The drawing under review shows one solid part. Ordinate dimensions are in mm from its lowest x, y, z. Round coordinates to 2 decimals unless told otherwise and drop trailing zeros. Write each loop counter-clockwise with the first axis right and the second up, starting at its lowest first coordinate (ties: lowest second). Pieces come first, ordered by that corner, then holes.
Item 1: Clearance check with flat-ended pins moving along their axes: pin 1 Ø1.5 at (x, y) = (11.5, 10) entering from +Z; pin 2 Ø1 at (x, y) = (15, 17) entering from +Z; pin 3 Ø4 at (y, z) = (7, 32.5) entering from +X. State where each tip first meets the part, or that it passes through.
Item 2: Add section A-A (x = 13.5). Give the boundary of the cut face in (y, z).
Item 3: Add section B-B (y = 8.5). Give the boundary of the cut face in (x, z) (1 decimal).
Item 4: To check wall thickness, follow L1, parallel to Y at x = 9, z = 10 (1 decimal); L2, parallel to Y at x = 5.25, z = 62.5; L3, parallel to X at y = 13.75, z = 27. State the ranges of each line that lie inside material, in increasing order.
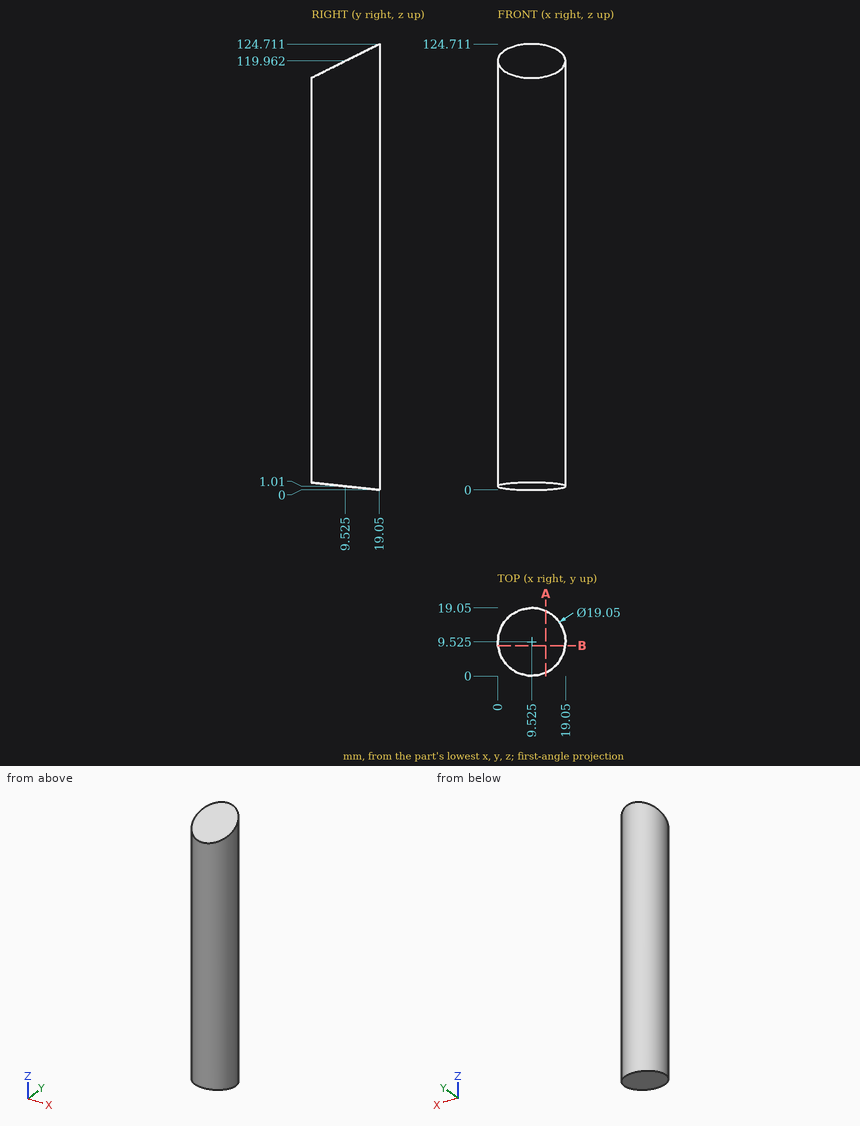
Numbers:
1. pin 1: stops at z = 120.57
1. pin 2: stops at z = 123.92
1. pin 3: stops at x = 19.04
2. outline: (0.87, 1.93) - (18.18, 0.09) - (18.18, 124.28) - (0.87, 115.65) - close
3. outline: (0.1, 1.1) - (19, 1.1) - (19, 119.5) - (0.1, 119.5) - close
4. L1: y = 0 to 19
4. L2: y = 1.01 to 18.04
4. L3: x = 0.99 to 18.06
